from build123d import *

# Parameters (mm, degrees)
SKETCH_R        = 3.8
PAD_DEPTH       = 3
PAD001_DEPTH    = 13
SKETCH002_R     = 4.3
POCKET_DEPTH    = 16.001
POCKET001_DEPTH = 9
SKETCH004_R     = 2.8
POCKET002_DEPTH = 20.001


with BuildPart() as part:
    # Sketch → Pad (new body)
    with BuildSketch(Plane.XY):
        with BuildLine():
            ThreePointArc((0, 5), (-5, 0), (0, -5))
            Line((0, -5), (25, -5))
            ThreePointArc((25, -5), (30, 0), (25, 5))
            Line((0, 5), (25, 5))
        make_face()
        Circle(SKETCH_R, mode=Mode.SUBTRACT)
        with Locations((25, 0)):
            Circle(SKETCH_R, mode=Mode.SUBTRACT)
    extrude(amount=PAD_DEPTH)

    # Sketch001 (on Face8 of Pad) → Pad001 (join)
    with BuildSketch(Plane.XY.offset(3)):
        with BuildLine():
            ThreePointArc((0, 5), (-5, 0), (0, -5))
            Line((0, -5), (25, -5))
            ThreePointArc((25, -5), (30, 0), (25, 5))
            Line((0, 5), (25, 5))
        make_face()
    extrude(amount=PAD001_DEPTH)

    # Sketch002 (on Face14 of Pad001) → Pocket (cut, through all)
    with BuildSketch(Plane.XY.offset(16)):
        with Locations((12.5, 0)):
            Circle(SKETCH002_R)
    extrude(amount=-POCKET_DEPTH, mode=Mode.SUBTRACT)

    # Sketch003 (on Face13 of Pocket) → Pocket001 (cut)
    with BuildSketch(Plane.XY.offset(16)):
        Polygon((18, 4.25), (22.5, 4.25), (22.5, -4.25), (18, -4.25), (18, 0), align=None)
        with BuildLine():
            Line((25, 0), (25, 5))
            ThreePointArc((25, -5), (30, 0), (25, 5))
            Line((25, -5), (25, 0))
        make_face()
    extrude(amount=-POCKET001_DEPTH, mode=Mode.SUBTRACT)

    # Sketch004 → Pocket002 (cut, through all)
    with BuildSketch(Plane.YZ.offset(10)):
        with Locations((0, 12)):
            Circle(SKETCH004_R)
    extrude(amount=POCKET002_DEPTH, mode=Mode.SUBTRACT)


solid = part.part
Can you work these out from the model? Positions are in its coordinate system, mm. A direction names the side the tool comes from. Give positions to 0.01 mm unless a question says otherwise; leave off trailing zeros. Write each loop counter-clockwise with the first axis right and the second up, starting at its lowest first coordinate (ties: lowest second). Pieces come first, ordered by that corner, then holes. Notation, with made-up numbers: (32, 75) -> (59, 75) arc R15 ccw to (59, 97) -> close; hole circle Ø9 at (7, -28). An arc over 180 degrees is marked (long way). Answer as a JSON object with one key per item and string values. Group by question number.
Item 1: Please list where these lines run through material, in increasing order: line 1 (Y direction, x = 12.5, z = 8); line 2 (X direction, y = 2.75, z = 13); line 3 (Y direction, x = 25, z = 0.75). Write a range as [from, to].
Item 2: I'm going to push flat-ended pins straight in: P1, Ø4, axis at y = 1.5, z = 8, coming from the -X side; P2, Ø1.5, axis at y = -2, z = 14, coming from the +X side; P3, Ø1.3, axis at x = 21, y = 0, coming from the +Z side; P4, Ø2.5, axis at y = 0, z = 13, coming from the +X side. Where does each tip first touch, or does it pass through?
Item 3: For faces 1 (the face through (23.732, -0.365, 14.776)), 2 (the face through (22.2, 2.57, 1.48)), 3 (the face through (20, 0, 7)), which set-ups out of +Z, -Z, +X, -X, +Y, -Y let a thin tool reach every point of the face, with its end or its side?
Item 4: Suppose I cut it at C-C (y = -1). State how many separate pieces and enclosed holes the cut face has, plus the area to 3 significant figures.
Item 5: Suppose I cut it at D-D (z = 4.5). Please give me the cut outline in (x, y).
Item 6: Suppose I cut it at A-A (z = 7.75). Please give me the cut outline in (x, y).
Item 7: Suppose I cut it at B-B (x = 12.5). Please give me the cut outline in (y, z), plus the area to 3 significant figures.
Item 8: We'd pull the mould along Y, two halves only. Please class faces 4 (the face through (25, 0, 9)), 5 (the face through (20, -4.25, 12)), 6 (the face through (30, 0, 3)), 7 (the face through (20, 4.25, 12)): +Y half, -Y half, draft (parallel to the pull), parting line (faces both ways), or undercut.
Findings:
{
 "1": {"line 1": "y = [-5, -4.3], [4.3, 5]", "line 2": "x = [-4.18, 9.19], [15.81, 18], [22.5, 25]", "line 3": "y = [-5, -3.8], [3.8, 5]"},
 "2": {"P1": "stops at x = -5", "P2": "stops at x = 25", "P3": "stops at z = 7", "P4": "stops at x = 8.39"},
 "3": {"face 1": "+X", "face 2": "-Z", "face 3": "+Z"},
 "4": {"separate pieces": "4", "enclosed holes": "0", "area": "274 mm²"},
 "5": {"outline": "(0, -5) -> (25, -5) arc R5 ccw to (25, 5) -> (0, 5) arc R5 ccw to start; hole circle Ø8.6 at (12.5, 0)"},
 "6": {"outline": "(0, -5) -> (25, -5) -> (25, 5) -> (0, 5) arc R5 ccw to start; hole circle Ø8.6 at (12.5, 0); hole (18, -4.25) -> (22.5, -4.25) -> (22.5, 4.25) -> (18, 4.25) -> close"},
 "7": {"outline": "(-5, 0) -> (-4.3, 0) -> (-4.3, 16) -> (-5, 16) -> close; (4.3, 0) -> (5, 0) -> (5, 16) -> (4.3, 16) -> close", "area": "22.4 mm²"},
 "8": {"face 4": "draft", "face 5": "undercut", "face 6": "parting line", "face 7": "undercut"}
}
